from build123d import *

# Parameters (mm, degrees)
F0_R     = 1.6
F1_DEPTH = 3.175


with BuildPart() as f1:
    # F0 (on Top) → F1 (new body)
    with BuildSketch(Plane.XY):
        with BuildLine():
            ThreePointArc((0, 6.35), (1.859872, 1.859872), (6.35, 0))
            Line((6.35, 0), (143.65, 0))
            ThreePointArc((143.65, 0), (148.140128, 1.859872), (150, 6.35))
            Line((150, 6.35), (150, 103.65))
            ThreePointArc((150, 103.65), (148.140128, 108.140128), (143.65, 110))
            Line((143.65, 110), (6.35, 110))
            ThreePointArc((6.35, 110), (1.859872, 108.140128), (0, 103.65))
            Line((0, 103.65), (0, 6.35))
        make_face()
        with Locations((5, 5)):
            Circle(F0_R, mode=Mode.SUBTRACT)
        with Locations((15, 5)):
            Circle(F0_R, mode=Mode.SUBTRACT)
        with Locations((25, 5)):
            Circle(F0_R, mode=Mode.SUBTRACT)
        with Locations((35, 5)):
            Circle(F0_R, mode=Mode.SUBTRACT)
        with Locations((5, 15)):
            Circle(F0_R, mode=Mode.SUBTRACT)
        with Locations((15.31, 17.535)):
            Circle(F0_R, mode=Mode.SUBTRACT)
        with Locations((5, 25)):
            Circle(F0_R, mode=Mode.SUBTRACT)
        with Locations((45, 5)):
            Circle(F0_R, mode=Mode.SUBTRACT)
        with Locations((55, 5)):
            Circle(F0_R, mode=Mode.SUBTRACT)
        with Locations((65, 5)):
            Circle(F0_R, mode=Mode.SUBTRACT)
        with Locations((5, 35)):
            Circle(F0_R, mode=Mode.SUBTRACT)
        with Locations((5, 45)):
            Circle(F0_R, mode=Mode.SUBTRACT)
        with Locations((75, 5)):
            Circle(F0_R, mode=Mode.SUBTRACT)
        with Locations((85, 5)):
            Circle(F0_R, mode=Mode.SUBTRACT)
        with Locations((95, 5)):
            Circle(F0_R, mode=Mode.SUBTRACT)
        with Locations((105, 5)):
            Circle(F0_R, mode=Mode.SUBTRACT)
        with Locations((115, 5)):
            Circle(F0_R, mode=Mode.SUBTRACT)
        with Locations((125, 5)):
            Circle(F0_R, mode=Mode.SUBTRACT)
        with Locations((135, 5)):
            Circle(F0_R, mode=Mode.SUBTRACT)
        with Locations((145, 5)):
            Circle(F0_R, mode=Mode.SUBTRACT)
        with Locations((134.69, 17.535)):
            Circle(F0_R, mode=Mode.SUBTRACT)
        with Locations((145, 15)):
            Circle(F0_R, mode=Mode.SUBTRACT)
        with Locations((145, 25)):
            Circle(F0_R, mode=Mode.SUBTRACT)
        with Locations((145, 35)):
            Circle(F0_R, mode=Mode.SUBTRACT)
        with Locations((145, 45)):
            Circle(F0_R, mode=Mode.SUBTRACT)
        with Locations((5, 55)):
            Circle(F0_R, mode=Mode.SUBTRACT)
        with Locations((5, 65)):
            Circle(F0_R, mode=Mode.SUBTRACT)
        with Locations((5, 75)):
            Circle(F0_R, mode=Mode.SUBTRACT)
        with Locations((5, 85)):
            Circle(F0_R, mode=Mode.SUBTRACT)
        with Locations((5, 95)):
            Circle(F0_R, mode=Mode.SUBTRACT)
        with Locations((14.04, 93.735)):
            Circle(F0_R, mode=Mode.SUBTRACT)
        with Locations((5, 105)):
            Circle(F0_R, mode=Mode.SUBTRACT)
        with Locations((15, 105)):
            Circle(F0_R, mode=Mode.SUBTRACT)
        with Locations((25, 105)):
            Circle(F0_R, mode=Mode.SUBTRACT)
        with Locations((35, 105)):
            Circle(F0_R, mode=Mode.SUBTRACT)
        with Locations((45, 105)):
            Circle(F0_R, mode=Mode.SUBTRACT)
        with Locations((55, 105)):
            Circle(F0_R, mode=Mode.SUBTRACT)
        with Locations((65, 105)):
            Circle(F0_R, mode=Mode.SUBTRACT)
        Polygon((20.31, 22.535), (10, 22.535), (10, 87.465), (20.31, 87.465), (20.31, 100), (129.69, 100), (129.69, 87.465), (140, 87.465), (140, 22.535), (129.69, 22.535), (129.69, 10), (20.31, 10), align=None, mode=Mode.SUBTRACT)
        with Locations((145, 55)):
            Circle(F0_R, mode=Mode.SUBTRACT)
        with Locations((145, 65)):
            Circle(F0_R, mode=Mode.SUBTRACT)
        with Locations((145, 75)):
            Circle(F0_R, mode=Mode.SUBTRACT)
        with Locations((75, 105)):
            Circle(F0_R, mode=Mode.SUBTRACT)
        with Locations((85, 105)):
            Circle(F0_R, mode=Mode.SUBTRACT)
        with Locations((95, 105)):
            Circle(F0_R, mode=Mode.SUBTRACT)
        with Locations((105, 105)):
            Circle(F0_R, mode=Mode.SUBTRACT)
        with Locations((145, 85)):
            Circle(F0_R, mode=Mode.SUBTRACT)
        with Locations((134.69, 92.465)):
            Circle(F0_R, mode=Mode.SUBTRACT)
        with Locations((145, 95)):
            Circle(F0_R, mode=Mode.SUBTRACT)
        with Locations((115, 105)):
            Circle(F0_R, mode=Mode.SUBTRACT)
        with Locations((125, 105)):
            Circle(F0_R, mode=Mode.SUBTRACT)
        with Locations((135, 105)):
            Circle(F0_R, mode=Mode.SUBTRACT)
        with Locations((145, 105)):
            Circle(F0_R, mode=Mode.SUBTRACT)
    extrude(amount=F1_DEPTH)


solid = f1.part
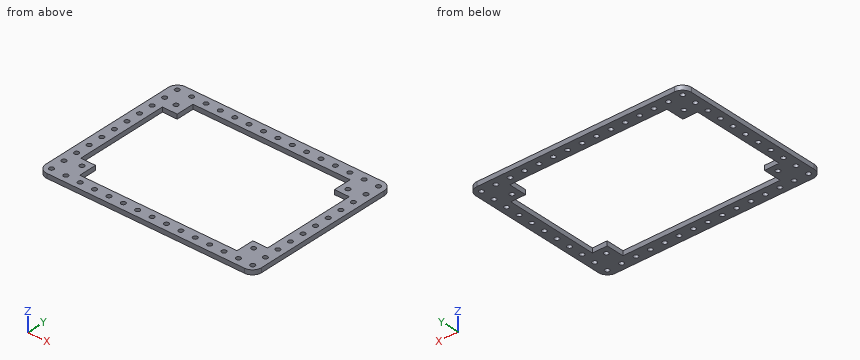
Build history of the part. All positions in model axes, mm. Coordinates: 2 decimals unless noted, no trailing zeros. Order: outer loops, then holes, each group sorted by start corner. A loop starts at its lowest first (then second) coordinate and runs counter-clockwise, first axis right, second up. Notation, with made-up numbers: (-26.75, 76.5) - (9.25, 76.5) arc R25 cw to (9.25, 95.5) - close; hole circle Ø4 at (66.25, 85). An arc over 180 degrees is marked (long way). Write each question's results on one line, items separated by ' | '. Start each with the question number.
Item 1: Wall check: probe 1 along X at (y, z) = (71.5, 2.45); probe 2 along Y at (x, z) = (31.5, 0.35); probe 3 along Y at (x, z) = (64, 2.65). Give the ranges that are in metal, low to high. Write a range as [from, to].
Item 2: Band-saw the part on A-A on x = 115. Write the cut outline in (y, z) (3 decimals), and give its area (3 significant figures).
Item 3: Flat gauge pin, fed straight in: pin 1 (1.9 mm diameter, centred on x = 115, y = 105, fed in from +Z). Where does the tip first touch, or does it go through?
Item 4: Band-saw the part on B-B on y = 85. Write the cut outline in (x, z) (3 decimals).
Item 5: Band-saw the part on C-C on z = 1.15. State how many separate pieces and enclosed holes the cut face has, and give its area (3 significant figures).
Numbers:
1) probe 1: [0, 10], [140, 150] | probe 2: [0, 10], [100, 110] | probe 3: [0, 3.75], [6.25, 10], [100, 103.75], [106.25, 110]
2) outline: (0, 0) - (3.4, 0) - (3.4, 3.175) - (0, 3.175) - close; (6.6, 0) - (10, 0) - (10, 3.175) - (6.6, 3.175) - close; (100, 0) - (103.4, 0) - (103.4, 3.175) - (100, 3.175) - close; (106.6, 0) - (110, 0) - (110, 3.175) - (106.6, 3.175) - close | area: 43.2 mm^2
3) pin 1: through
4) outline: (0, 0) - (3.4, 0) - (3.4, 3.175) - (0, 3.175) - close; (6.6, 0) - (10, 0) - (10, 3.175) - (6.6, 3.175) - close; (140, 0) - (143.4, 0) - (143.4, 3.175) - (140, 3.175) - close; (146.6, 0) - (150, 0) - (150, 3.175) - (146.6, 3.175) - close
5) separate pieces: 1 | enclosed holes: 53 | area: 4,860 mm^2
